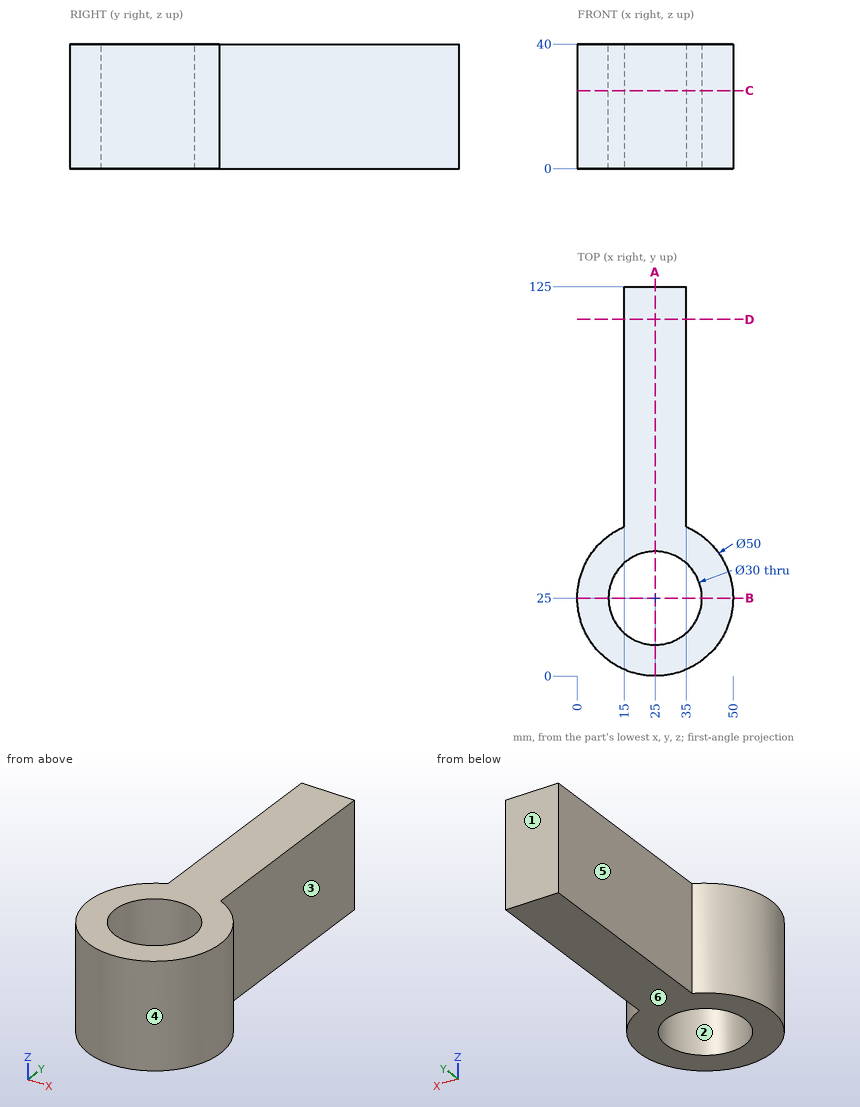
Check sheet for the drawn part. Datum: minimum x, y, z corner. Units: mm. A direction names the side the tool comes from. Round coordinates to 2 decimals unless told otherwise and drop trailing zeros. Loops run counter-clockwise (first coordinate to the right, second up) from the corner with the lowest first, then second, coordinate; pieces in that order, holes last. Notation, with made-up numbers: (-1, -1) - (36, -1) arc R20 cw to (36, 23) - close; hole circle Ø6 at (-28, -19.75). An arc over 180 degrees is marked (long way). Write each question's results on one line, items separated by ' | '. Start each with the question number.
Q1. Gauge pin test, flat ends, axial feed: P1, Ø10, axis at x = 20, y = 49, coming from the -Z side; P2, Ø1.5, axis at x = 18, z = 8.5, coming from the -Y side; P3, Ø24, axis at x = 25, y = 25, coming from the -Z side; P4, Ø3, axis at x = 21, z = 13.5, coming from the -Y side. Record the tip position at first contact, or that the pin passes through.
Q2. Cross-section at A-A on x = 25. Enter the section's corners in (y, z).
Q3. Cross-section at C-C on z = 25. Enter the section's corners in (x, y).
Q4. Cross-section at D-D on y = 114.5. Enter the section's corners in (x, z).
Q5. Thickness scan on line 1 (Y direction, x = 25, z = 21); line 2 (X direction, y = 63, z = 12); line 3 (Y direction, x = 29, z = 6.5). Record the ranges inside material, lowest first. Write a range as [from, to].
Q6. Release check for a two-part mould opening along Y. For the marked faces 1, 2, 3 and 4 record: +Y half, -Y half, draft (parallel to the pull), parting line (faces both ways), or undercut.
Q7. Cross-section at B-B on y = 25. Enter the section's corners in (x, z).
Q8. Access from +Z, -Z, +X, -X, +Y, -Y to the whole of each face (thin tool, end or side, straight path). Record for the marked faces 5 and 6.
Answers below:
1) P1: stops at z = 0 | P2: stops at y = 0.79 | P3: passes through | P4: stops at y = 0.13
2) outline: (0, 0) - (10, 0) - (10, 40) - (0, 40) - close; (40, 0) - (125, 0) - (125, 40) - (40, 40) - close
3) outline: (15, 47.91) arc R25 ccw (long way) to (35, 47.91) - (35, 125) - (15, 125) - close; hole circle Ø30 at (25, 25)
4) outline: (15, 0) - (35, 0) - (35, 40) - (15, 40) - close
5) line 1: y = [0, 10], [40, 125] | line 2: x = [15, 35] | line 3: y = [0.32, 10.54], [39.46, 125]
6) face 1: +Y half | face 2: undercut | face 3: draft | face 4: parting line
7) outline: (0, 0) - (10, 0) - (10, 40) - (0, 40) - close; (40, 0) - (50, 0) - (50, 40) - (40, 40) - close
8) face 5: +Z, -Z, -X, +Y | face 6: -Z, +X, -X, +Y, -Y
